```python
from build123d import *

# Parameters (mm, degrees)
SKETCH_1_W          = 20
SKETCH_1_H          = 15
EXTRUDE_1_DEPTH     = 20
SKETCH_2_W          = 7
SKETCH_2_H          = 15
EXTRUDE_6_DEPTH     = 4
EXTRUDE_7_DEPTH     = 1.5
SKETCH_10_R         = 1.5
CUT_EXTRUDE_4_DEPTH = 1.5
FILLET_1_R          = 4
SKETCH_11_R         = 4.05
CUT_EXTRUDE_5_DEPTH = 13
CUT_EXTRUDE_6_DEPTH = 10


with BuildPart() as part:
    # 草图1 → 凸台-拉伸1 (new body)
    with BuildSketch(Plane.XY):
        Rectangle(SKETCH_1_W, SKETCH_1_H)
    extrude(amount=EXTRUDE_1_DEPTH)

    # 草图2 → 凸台-拉伸6 (add)
    # profile 1 of 2: a face of its own
    with BuildSketch(Plane.XY):
        with Locations((-13.5, 0)):
            Rectangle(SKETCH_2_W, SKETCH_2_H)
        Polygon((-10.1, 0), (-11.8, 2.944486373), (-15.2, 2.944486373), (-16.9, 0), (-15.2, -2.944486373), (-11.8, -2.944486373), align=None, mode=Mode.SUBTRACT)
    # profile 2 of 2: a face of its own
    with BuildSketch(Plane.XY):
        with Locations((13.5, 0)):
            Rectangle(SKETCH_2_W, SKETCH_2_H)
        Polygon((16.9, 0), (15.2, 2.944486373), (11.8, 2.944486373), (10.1, 0), (11.8, -2.944486373), (15.2, -2.944486373), align=None, mode=Mode.SUBTRACT)
    extrude(amount=EXTRUDE_6_DEPTH)

    # 草图9 → 凸台-拉伸7 (add)
    with BuildSketch(Plane(origin=(0, 0, 0), x_dir=(-1, 0, 0), z_dir=(0, 0, -1))):
        Polygon((-10.1, 0), (-11.8, 2.944486373), (-15.2, 2.944486373), (-16.9, 0), (-15.2, -2.944486373), (-11.8, -2.944486373), align=None)
        Polygon((16.9, 0), (15.2, 2.944486373), (11.8, 2.944486373), (10.1, 0), (11.8, -2.944486373), (15.2, -2.944486373), align=None)
    extrude(amount=-EXTRUDE_7_DEPTH)

    # 草图10 → 切除-拉伸4 (cut)
    with BuildSketch(Plane(origin=(0, 0, 0), x_dir=(-1, 0, 0), z_dir=(0, 0, -1))):
        with Locations((-13.5, 0)):
            Circle(SKETCH_10_R)
        with Locations((13.5, 0)):
            Circle(SKETCH_10_R)
    extrude(amount=-CUT_EXTRUDE_4_DEPTH, mode=Mode.SUBTRACT)

    # 圆角1
    fillet_1_edges = [part.edges().sort_by_distance(p)[0] for p in [
        (-17, 7.5, 2),
        (-17, -7.5, 2),
        (17, -7.5, 2),
        (17, 7.5, 2),
    ]]
    fillet(fillet_1_edges, radius=FILLET_1_R)

    # 草图11 → 切除-拉伸5 (cut)
    with BuildSketch(Plane(origin=(0, 13.321067812, 13.321067812), x_dir=(1, 0, 0), z_dir=(0, 0.7071067811865389, 0.7071067811865561))):
        with Locations(Location((1, -10.445436483, 0), (0, 0, 270))):
            Circle(SKETCH_11_R)
    extrude(amount=-CUT_EXTRUDE_5_DEPTH, mode=Mode.SUBTRACT)

    # 草图12 → 切除-拉伸6 (cut)
    with BuildSketch(Plane(origin=(0, 13.321067812, 13.321067812), x_dir=(1, 0, 0), z_dir=(0, -0.7071067811865389, -0.7071067811865562))):
        Polygon((4.391788695, 8.232233047), (-2.391788695, 8.232233047), (-2.708147576, 8.816896782), (-2.924601891, 9.445436483), (4.924601891, 9.445436483), (4.643673318, 8.677345775), align=None)
    extrude(amount=-CUT_EXTRUDE_6_DEPTH, mode=Mode.SUBTRACT)


solid = part.part
```
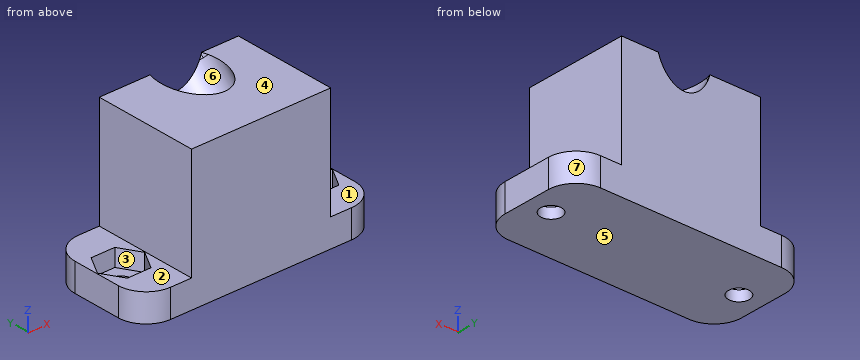
Here's how the part is built. I have some questions about the finished solid (model axes, mm). Face numbers are marked on the shaded views. A direction names the side the tool comes from. Give positions to 0.01 mm unless a question says otherwise; leave off trailing zeros. Write each loop counter-clockwise with the first axis right and the second up, starting at its lowest first coordinate (ties: lowest second). Pieces come first, ordered by that corner, then holes. Notation, with made-up numbers: M 78.25,13.5 L 118.25,13.5 A19 ccw 118.25,17.5 Z; hole C -39.75,19 d10. An arc over 180 degrees is marked long. Put each result on its own line as item: value. Start each with the question number.
Item 1: Will these pins go through, and if not, where does the flat tip stop? pin 1 (4.5 mm diameter, centred on x = -12, y = -1, fed in from +Z); pin 2 (4.5 mm diameter, centred on y = 2.5, z = 12, fed in from -X); pin 3 (3.5 mm diameter, centred on x = -13.5, y = 3.5, fed in from +Z); pin 4 (3 mm diameter, centred on x = 13, y = 0.5, fed in from +Z).
Item 2: If we section it at C-C, the plane y = 1: Count the separate pieces of the cut face and the enclosed holes in it, then the cut area to 3 significant figures.
Item 3: If we section it at A-A, the plane x = 13.5: Write out the boundary of the cut face in (y, z), then the cut area to 3 significant figures.
Item 4: On a 3-axis mill with a long thin cutter (end or side, diameter ignored), from which of +Z, -Z, +X, -X, +Y, -Y can I reach the whole of each face in a straight line? I mean the marked faces 1, 2 and 3. Say none if no direction works.
Item 5: Thinking about a two-plate mould opening in Z: for the marked faces 4, 5, 6 and 7, which applies, +Z half, -Z half, draft (parallel to the pull), parting line (faces both ways), or undercut?
Item 6: If we section it at B-B, the plane z = 7.5: Write out the boundary of the cut face in (x, y).
Item 7: I need wall thicknesses on L1, parallel to Y at x = 13, z = 1.75; L2, parallel to Z at x = -11.5, y = -0.25; L3, parallel to X at y = -6, z = 16.25. Which ranges of each line are inside material? Lowest first, please. Write a range as from..to.
Values:
1. pin 1: z = 20
1. pin 2: x = -10
1. pin 3: z = 4
1. pin 4: z = 1.5
2. separate pieces: 3
2. enclosed holes: 0
2. area: 354 mm²
3. outline: M -7.47,0 L -1.5,0 L -1.5,1.5 L -2.94,1.5 L -2.94,4 L -7.47,4 Z; M 1.5,0 L 7.47,0 L 7.47,4 L 2.94,4 L 2.94,1.5 L 1.5,1.5 Z
3. area: 40.5 mm²
4. face 1: +Z, +X, +Y, -Y
4. face 2: +Z, -X, +Y, -Y
4. face 3: +Z
5. face 4: +Z half
5. face 5: -Z half
5. face 6: undercut
5. face 7: draft
6. outline: M -10,-7.5 L 10,-7.5 L 10,7.5 L -10,7.5 Z
7. L1: -7.5..-2.94, 2.94..7.5
7. L2: 0..1.5
7. L3: -10..10
